The listing builds one solid part. Answer for the finished solid, in the listing's coordinates (mm). A direction names the side the tool comes from. Coordinates: 2 decimals unless noted, no trailing zeros. Loops run counter-clockwise (first coordinate to the right, second up) from the corner with the lowest first, then second, coordinate; pieces in that order, holes last. Notation, with made-up numbers: (77, -26) -> (94, -26) arc R24 cw to (94, -9) -> close; hole circle Ø6 at (15, -27.75). An arc over 180 degrees is marked (long way). Answer in a Markdown table with one row per item.
```python
from build123d import *

# Parameters (mm, degrees)
BOSS_EXTRUDE1_DEPTH = 3
FILLET1_R           = 0.2


with BuildPart() as part:
    # Sketch1 → Boss-Extrude1 (new body)
    with BuildSketch(Plane(origin=(0, 0, 0), x_dir=(1, 0, 0), z_dir=(0, 1, 0))):
        with BuildLine():
            Line((10, 0), (-10, 0))
            Line((-10, 0), (-10, 6))
            ThreePointArc((-10, 6), (-11.5, 7.5), (-13, 6))
            Line((-13, 6), (-13, 0))
            Line((-13, 0), (-33, 0))
            ThreePointArc((-33, 0), (-34.414213562, 0.585786438), (-35, 2))
            Line((-35, 2), (-35, 9.156613858))
            ThreePointArc((-35, 9.156613858), (-34.763762616, 9.802111083), (-34.166666667, 10.142627155))
            ThreePointArc((-34.166666667, 10.142627155), (0, 13.009901233), (34.166666667, 10.142627155))
            ThreePointArc((34.166666667, 10.142627155), (34.763762616, 9.802111083), (35, 9.156613858))
            Line((35, 9.156613858), (35, 2))
            ThreePointArc((35, 2), (34.414213562, 0.585786438), (33, 0))
            Line((33, 0), (13, 0))
            Line((13, 0), (13, 6))
            ThreePointArc((13, 6), (11.5, 7.5), (10, 6))
            Line((10, 6), (10, 0))
        make_face()
    extrude(amount=BOSS_EXTRUDE1_DEPTH)

    # Fillet1
    fillet1_edges = [part.edges().sort_by_distance(p)[0] for p in [
        (10, 3, -3),
        (11.5, 3, -7.5),
        (-11.5, 0, -7.5),
        (-13, 0, -3),
        (-23, 0, 0),
        (-34.414213562, 0, -0.585786438),
        (-35, 0, -5.578306929),
        (13, 3, -3),
        (-34.763762616, 0, -9.802111083),
        (0, 0, -13.009901233),
        (34.763762616, 0, -9.802111083),
        (35, 0, -5.578306929),
        (34.414213562, 0, -0.585786438),
        (23, 0, 0),
        (13, 0, -3),
        (11.5, 0, -7.5),
        (23, 3, 0),
        (10, 0, -3),
        (0, 0, 0),
        (-10, 0, -3),
        (34.414213562, 3, -0.585786438),
        (35, 3, -5.578306929),
        (-13, 1.5, 0),
        (13, 1.5, 0),
        (10, 1.5, 0),
        (-10, 1.5, 0),
        (34.763762616, 3, -9.802111083),
        (0, 3, -13.009901233),
        (-34.763762616, 3, -9.802111083),
        (-35, 3, -5.578306929),
        (-10, 3, -3),
        (-34.414213562, 3, -0.585786438),
        (-23, 3, 0),
        (-13, 3, -3),
        (-11.5, 3, -7.5),
        (0, 3, 0),
    ]]
    fillet(fillet1_edges, radius=FILLET1_R)


solid = part.part
```
Item 1: Determine the mould class of faces 3 (the face through (-13, 1, -3)), 4 (the face through (-35, 1, -6)), 5 (the face through (0, 0, -7)) for opening direction X: +X half, -X half, draft (parallel to the pull), parting line (faces both ways), or undercut.
Findings below:
| item | result |
|---|---|
| face 3 | undercut |
| face 4 | -X half |
| face 5 | draft |
Item 2: Find the intervals of material crossed by probe 1 along X at (y, z) = (2.05, -5.5); probe 2 along X at (y, z) = (1.1, -1.5); probe 3 along Z at (x, y) = (1, 1), in increasing order.
Findings below:
| item | result |
|---|---|
| probe 1 | x = -35 to -13, -10 to 10, 13 to 35 |
| probe 2 | x = -34.94 to -13, -10 to 10, 13 to 34.94 |
| probe 3 | z = -13.01 to 0 |
Item 3: A tool of negligible diameter and unlimited length cuts with its end or side. For faces 1 (the face through (13, 1, -3)), 2 (the face through (-0.48, 1.48, -13.01)), from which of +Z, -Z, +X, -X, +Y, -Y can it reach the whole face along a straight path? Write none if from no direction.
Findings below:
| item | result |
|---|---|
| face 1 | +Z, +Y, -Y |
| face 2 | -Z, +Y, -Y |
Item 4: A cutting plane is placed at B-B, the plane y = 2.15. Determine the outline of the cut face in (x, z).
Findings below:
| item | result |
|---|---|
| outline | (-35, -9.16) arc R1 ccw to (-34.17, -10.14) arc R205 ccw to (34.17, -10.14) arc R1 ccw to (35, -9.16) -> (35, -2) arc R2 ccw to (33, 0) -> (13.2, 0) arc R0.2 ccw to (13, -0.2) -> (13, -6) arc R1.5 cw to (10, -6) -> (10, -0.2) arc R0.2 ccw to (9.8, 0) -> (-9.8, 0) arc R0.2 ccw to (-10, -0.2) -> (-10, -6) arc R1.5 cw to (-13, -6) -> (-13, -0.2) arc R0.2 ccw to (-13.2, 0) -> (-33, 0) arc R2 ccw to (-35, -2) -> close |
Item 5: A cutting plane is placed at A-A, the plane z = -3. Determine the outline of the cut face in (x, y).
Findings below:
| item | result |
|---|---|
| outline | (-35, 0.2) arc R0.2 ccw to (-34.8, 0) -> (-13.2, 0) arc R0.2 ccw to (-13, 0.2) -> (-13, 2.8) arc R0.2 ccw to (-13.2, 3) -> (-34.8, 3) arc R0.2 ccw to (-35, 2.8) -> close; (-10, 0.2) arc R0.2 ccw to (-9.8, 0) -> (9.8, 0) arc R0.2 ccw to (10, 0.2) -> (10, 2.8) arc R0.2 ccw to (9.8, 3) -> (-9.8, 3) arc R0.2 ccw to (-10, 2.8) -> close; (13, 0.2) arc R0.2 ccw to (13.2, 0) -> (34.8, 0) arc R0.2 ccw to (35, 0.2) -> (35, 2.8) arc R0.2 ccw to (34.8, 3) -> (13.2, 3) arc R0.2 ccw to (13, 2.8) -> close |
